from build123d import *

# Parameters (mm, degrees)
SKETCH1_R           = 11.5
BOSS_EXTRUDE1_DEPTH = 65
SKETCH2_R           = 2
CUT_EXTRUDE1_DEPTH  = 10
BOSS_EXTRUDE2_START = 3
SKETCH3_R           = 4
SKETCH3_R_2         = 2
BOSS_EXTRUDE2_DEPTH = 3
FILLET1_R           = 3


with BuildPart() as part:
    # Sketch1 → Boss-Extrude1 (new body)
    with BuildSketch(Plane(origin=(0, 0, 0), x_dir=(1, 0, 0), z_dir=(0, 1, 0))):
        with BuildLine():
            Line((-28.353157483, 3), (123.274320599, 3))
            ThreePointArc((123.274320599, 3), (151.960581558, 0), (123.274320599, -3))
            Line((123.274320599, -3), (-28.353157483, -3))
            ThreePointArc((-28.353157483, -3), (-57.039418442, 0), (-28.353157483, 3))
        make_face()
        with Locations(Location((-42.539418442, 0, 0), (0, 0, 270))):
            Circle(SKETCH1_R, mode=Mode.SUBTRACT)
        with Locations(Location((137.460581558, 0, 0), (0, 0, 270))):
            Circle(SKETCH1_R, mode=Mode.SUBTRACT)
    extrude(amount=BOSS_EXTRUDE1_DEPTH)

    # Sketch2 → Cut-Extrude1 (cut)
    with BuildSketch(Plane.XY.offset(3)):
        with Locations((-13.353157483, 57)):
            Circle(SKETCH2_R)
        with Locations((-8.353157483, 9)):
            Circle(SKETCH2_R)
        with Locations((66.646842517, 9)):
            Circle(SKETCH2_R)
        with Locations((68.646842517, 57)):
            Circle(SKETCH2_R)
    extrude(amount=-CUT_EXTRUDE1_DEPTH, mode=Mode.SUBTRACT)

    # Sketch3 → Boss-Extrude2 (add)
    # profile 1 of 4: a face of its own
    with BuildSketch(Plane.XY.offset(3).offset(BOSS_EXTRUDE2_START)):
        with Locations(Location((-13.353157483, 57, 0), (0, 0, 180))):
            Circle(SKETCH3_R)
        with Locations((-13.353157483, 57)):
            Circle(SKETCH3_R_2, mode=Mode.SUBTRACT)
    # profile 2 of 4: a face of its own
    with BuildSketch(Plane.XY.offset(3).offset(BOSS_EXTRUDE2_START)):
        with Locations(Location((68.646842517, 57, 0), (0, 0, 180))):
            Circle(SKETCH3_R)
        with Locations((68.646842517, 57)):
            Circle(SKETCH3_R_2, mode=Mode.SUBTRACT)
    # profile 3 of 4: a face of its own
    with BuildSketch(Plane.XY.offset(3).offset(BOSS_EXTRUDE2_START)):
        with Locations(Location((-8.353157483, 9, 0), (0, 0, 180))):
            Circle(SKETCH3_R)
        with Locations((-8.353157483, 9)):
            Circle(SKETCH3_R_2, mode=Mode.SUBTRACT)
    # profile 4 of 4: a face of its own
    with BuildSketch(Plane.XY.offset(3).offset(BOSS_EXTRUDE2_START)):
        with Locations(Location((66.646842517, 9, 0), (0, 0, 180))):
            Circle(SKETCH3_R)
        with Locations((66.646842517, 9)):
            Circle(SKETCH3_R_2, mode=Mode.SUBTRACT)
    extrude(amount=-BOSS_EXTRUDE2_DEPTH)

    # Fillet1
    fillet1_edges = [part.edges().sort_by_distance(p)[0] for p in [
        (-9.353157483, 57, 3),
        (72.646842517, 57, 3),
        (-4.353157483, 9, 3),
        (70.646842517, 9, 3),
    ]]
    fillet(fillet1_edges, radius=FILLET1_R - 0.0001)  # a hair under: the kernel refuses the full size


solid = part.part
Can you work these out from the model? Positions are in its coordinate system, mm. A direction names the side the tool comes from. Round coordinates to 2 decimals unless told otherwise and drop trailing zeros. Loops run counter-clockwise (first coordinate to the right, second up) from the corner with the lowest first, then second, coordinate; pieces in that order, holes last. Notation, with made-up numbers: (4, -31.5) - (58, -31.5) arc R22 ccw to (58, -2.5) - close; hole circle Ø10 at (42.5, 38.25). An arc over 180 degrees is marked (long way). Answer in a Markdown table with one row per item. Add a question column.
Q1. I want a section at C-C on z = -8.5. List the corners of the cut face in (x, y) for me, and give its area (3 significant figures).
Q2. I want a section at B-B on y = 9. Count the separate pieces of the cut face and the enclosed holes in it, and give its area (3 significant figures).
Q3. Which directions (+Z, -Z, +X, -X, +Y, -Y) give clear straight access to the entire face, cutting with the end or side of a thin tool? Please do faces 4 (the flat face through (70, 55, 6)), 5 (the cylindrical face through (-57.027, 32.045, 0.595)), 6 (the flat face through (46, 32, -3)).
Q4. I want a section at A-A on z = 0. List the corners of the cut face in (x, y) for me, and give its area (3 significant figures).
Q5. For pin 1 Ø2.5 at (x, y) = (-7, 7.5) entering from +Z; pin 2 Ø2.5 at (x, y) = (-8.35, 9) entering from +Z; pin 3 Ø8 at (x, y) = (-16.5, 25) entering from -Z; pin 4 Ø6 at (x, z) = (-22.5, 1.5) entering from -Y, each with a flat end and sliding along its axis, tell me the tip position at first contact or that it passes through.
Q6. I need wall thicknesses on L1, parallel to Y at x = 67.5, z = -1.25; L2, parallel to X at y = 17, z = -4.5; L3, parallel to X at y = 61, z = -7.75. Which ranges of each line are inside material? Lowest first, please.
Q7. I want a section at D-D on x = 48.5. List the corners of the cut face in (y, z) for me.
Q8. We'd pull the mould along Y, two halves only. Please class faces 1 (the flat face through (56, 65, 0)), 2 (the cylindrical face through (-53.766, 32.045, -2.493)), 3 (the cylindrical face through (67.17, 58.35, 1.56)): pulls with the +Y half, pulls with the -Y half, needs draft (parallel to the pull), parting line crosses it, or undercut.
A:
| question | item | result |
|---|---|---|
| 1 | outline | (-54.29, 0) - (-50.29, 0) - (-50.29, 65) - (-54.29, 65) - close; (-34.79, 0) - (-30.79, 0) - (-30.79, 65) - (-34.79, 65) - close; (125.71, 0) - (129.71, 0) - (129.71, 65) - (125.71, 65) - close; (145.21, 0) - (149.21, 0) - (149.21, 65) - (145.21, 65) - close |
| 1 | area | 1,040 mm^2 |
| 2 | separate pieces | 3 |
| 2 | enclosed holes | 2 |
| 2 | area | 1,380 mm^2 |
| 3 | face 4 | +Z, +Y, -Y |
| 3 | face 5 | +Y, -Y |
| 3 | face 6 | -Z, +Y, -Y |
| 4 | outline | (-57.04, 0) - (-54.04, 0) - (-54.04, 65) - (-57.04, 65) - close; (-31.04, 0) - (125.96, 0) - (125.96, 65) - (-31.04, 65) - close; (148.96, 0) - (151.96, 0) - (151.96, 65) - (148.96, 65) - close; hole circle Ø4 at (-13.35, 57); hole circle Ø4 at (-8.35, 9); hole circle Ø4 at (66.65, 9); hole circle Ø4 at (68.65, 57) |
| 4 | area | 10,500 mm^2 |
| 5 | pin 1 | z = 6 |
| 5 | pin 2 | through |
| 5 | pin 3 | z = -3 |
| 5 | pin 4 | y = 0 |
| 6 | L1 | 0 to 7.19, 10.81 to 55.36, 58.64 to 65 |
| 6 | L2 | -56.32 to -53.12, -31.96 to -28.76, 123.68 to 126.88, 148.04 to 151.24 |
| 6 | L3 | -54.79 to -51.04, -34.04 to -30.28, 125.21 to 128.96, 145.96 to 149.72 |
| 7 | outline | (0, -3) - (65, -3) - (65, 3) - (0, 3) - close |
| 8 | face 1 | pulls with the +Y half |
| 8 | face 2 | needs draft |
| 8 | face 3 | undercut |
